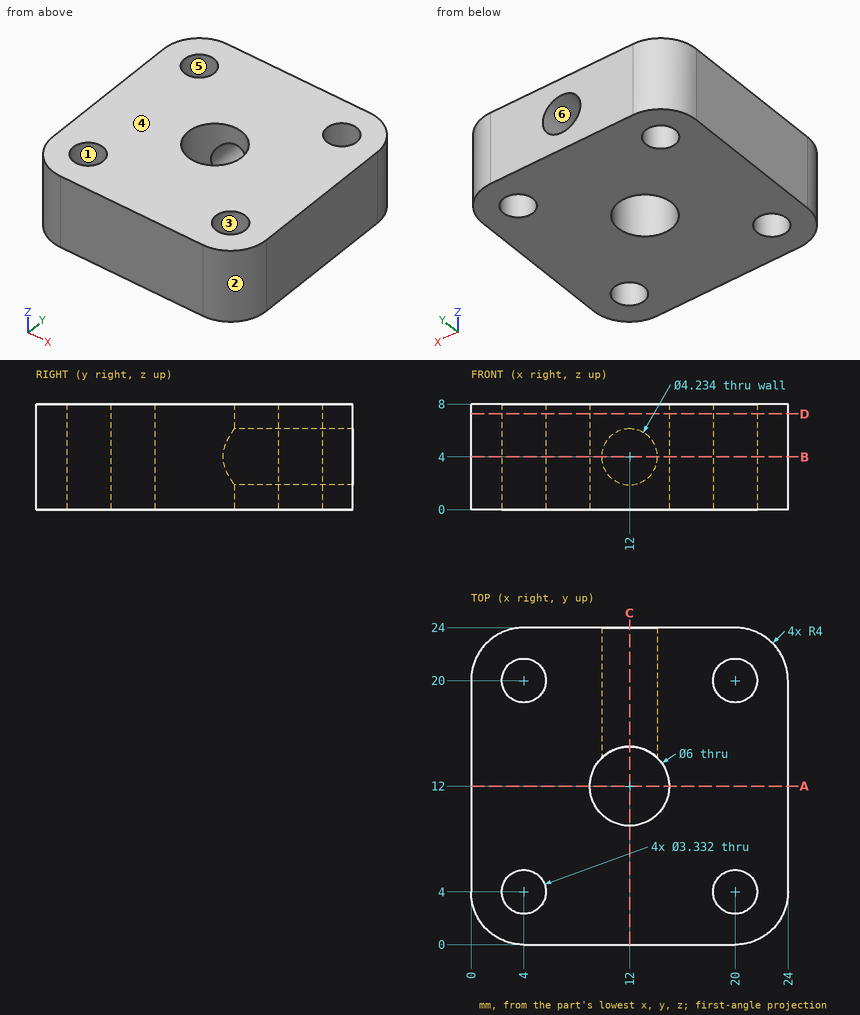
Print and shaded views of the part. All mm, measured from the part's lowest x, y and z. A direction names the side the tool comes from. Round coordinates to 2 decimals unless told otherwise and drop trailing zeros. Order: outer loops, then holes, each group sorted by start corner. A loop starts at its lowest first (then second) coordinate and runs counter-clockwise, first axis right, second up.
Q1. Which spindle directions (+Z, -Z, +X, -X, +Y, -Y) get a long thin tool onto all of the face, cutting with end or side? Do the marked faces 5 and 6. Say none if no direction does.
Q2. Wall check: L1, parallel to X at y = 4, z = 5; L2, parallel to X at y = 17.75, z = 4; L3, parallel to X at y = 20, z = 3.75. Give the ranges that are in metal, low to high.
Q3. Slice it at B-B (z = 4). Write the cut outline in (x, y), and give its area (3 significant figures).
Q4. Two-plate mould, pull along Y, no slides. Class the marked faces 1, 2, 3 and 4: pulls with the +Y half, pulls with the -Y half, needs draft (parallel to the pull), parting line crosses it, or undercut.
Q5. Drop a flat-ended pin along its axis: pin 1 (4 mm diameter, centred on y = 21, z = 5, fed in from -X). Give the stop position or say it passes through.
Q6. Slice it at D-D (z = 7.25). Write the cut outline in (x, y), and give its area (3 significant figures).
Q7. Slice it at C-C (x = 12). Write the cut outline in (y, z).
Q8. Slice it at A-A (y = 12). Write the cut outline in (x, z).
Results below:
1. face 5: +Z, -Z
1. face 6: +Y
2. L1: x = 0 to 2.33, 5.67 to 18.33, 21.67 to 24
2. L2: x = 0 to 9.88, 14.12 to 24
2. L3: x = 0 to 2.33, 5.67 to 9.9, 14.1 to 18.33, 21.67 to 24
3. outline: (0, 4) arc R4 ccw to (4, 0) - (20, 0) arc R4 ccw to (24, 4) - (24, 20) arc R4 ccw to (20, 24) - (14.12, 24) - (14.12, 14.13) arc R3 cw (long way) to (9.88, 14.13) - (9.88, 24) - (4, 24) arc R4 ccw to (0, 20) - close; hole circle Ø3.33 at (4, 4); hole circle Ø3.33 at (4, 20); hole circle Ø3.33 at (20, 4); hole circle Ø3.33 at (20, 20)
3. area: 460 mm2
4. face 1: undercut
4. face 2: pulls with the -Y half
4. face 3: undercut
4. face 4: needs draft
5. pin 1: stops at x = 0
6. outline: (0, 4) arc R4 ccw to (4, 0) - (20, 0) arc R4 ccw to (24, 4) - (24, 20) arc R4 ccw to (20, 24) - (4, 24) arc R4 ccw to (0, 20) - close; hole circle Ø3.33 at (4, 4); hole circle Ø3.33 at (4, 20); hole circle Ø6 at (12, 12); hole circle Ø3.33 at (20, 4); hole circle Ø3.33 at (20, 20)
6. area: 499 mm2
7. outline: (0, 0) - (9, 0) - (9, 8) - (0, 8) - close; (15, 0) - (24, 0) - (24, 1.88) - (15, 1.88) - close; (15, 6.12) - (24, 6.12) - (24, 8) - (15, 8) - close
8. outline: (0, 0) - (9, 0) - (9, 8) - (0, 8) - close; (15, 0) - (24, 0) - (24, 8) - (15, 8) - close
